The model under review builds one solid part; all positions refer to its coordinate system, in mm. A direction names the side the tool comes from. Round coordinates to 2 decimals unless told otherwise and drop trailing zeros. Order: outer loops, then holes, each group sorted by start corner. A loop starts at its lowest first (then second) coordinate and runs counter-clockwise, first axis right, second up. Notation, with made-up numbers: M -35.5,35.5 L 7.5,35.5 A15 cw 7.5,58.5 Z; hole C 83.25,86 d8. An arc over 180 degrees is marked long. One line per item, written item: value. Start each with the question number.
Autodesk Inventor part; units mm, degrees
ref_plane "YZ Plane" through (0, 0, 0) normal (1, 0, 0) x (0, 1, 0)
ref_plane "XZ Plane" through (0, 0, 0) normal (0, 1, 0) x (-1, 0, 0)
ref_plane "XY Plane" through (0, 0, 0) normal (0, 0, 1) x (1, 0, 0)
sketch "Sketch1" plane through (0, 0, 0) normal (1, 0, 0) x (0, 1, 0)
  line L0 (15.7193, -14.4333) -> (-9.6807, -14.4333)
  line L1 (-9.6807, -14.4333) -> (-9.6807, 10.9667)
  line L2 (-9.6807, 10.9667) -> (15.7193, 10.9667)
  line L3 (15.7193, 10.9667) -> (15.7193, -14.4333)
  line L4 (15.7193, -14.4333) -> (-9.6807, 10.9667) construction
  line L5 (-9.6807, -14.4333) -> (15.7193, 10.9667) construction
  point P0 (0, 0)
  point P1 (3.0193, -1.7333)
  dimension "d0" = 25.4
  dimension "d1" = 25.4
extrude "Extrusion1" add sketch "Sketch1" along normal blind 25.4
sketch "Sketch2" plane through (0, -9.6807, 10.9667) normal (0, 0, 1) x (1, 0, 0)
  circle A0 centre (12.7, 12.7) radius 2.3749
  point P0 (0, 9.6807)
  dimension "d4" = 4.7498
sketch "Sketch3" plane through (0, -9.6807, 10.9667) normal (0, 0, 1) x (1, 0, 0)
  line L0 (0, 0) -> (0, 25.4)
  line L1 (0, 0) -> (25.4, 0)
  line L2 (25.4, 25.4) -> (25.4, 0)
  line L3 (0, 25.4) -> (25.4, 25.4)
  point P0 (0, 9.6807)
extrude "Extrusion2" cut sketch "Sketch2" against normal blind 1.27
sketch "Sketch4" plane through (0, 15.7193, 10.9667) normal (0, 1, 0) x (1, 0, 0)
  circle A0 centre (6.3453, 19.0547) radius 2.3749
  circle A1 centre (12.7, 12.7) radius 2.3749
  circle A2 centre (19.0547, 6.3453) radius 2.3749
  point P0 (0, 10.9667)
  dimension "d7" = 4.7498
  dimension "d8" = 4.7498
  dimension "d9" = 4.7498
extrude "Extrusion3" cut sketch "Sketch4" against normal blind 1.27
sketch "Sketch5" plane through (0, -9.6807, -14.4333) normal (0, -1, 0) x (1, 0, 0)
  circle A0 centre (6.3453, 19.0547) radius 2.3749
  circle A1 centre (19.0547, 19.0547) radius 2.3749
  circle A2 centre (6.3453, 6.3453) radius 2.3749
  circle A3 centre (19.0547, 6.3453) radius 2.3749
  point P0 (0, 14.4333)
  dimension "d12" = 4.7498
  dimension "d13" = 4.7498
  dimension "d14" = 4.7498
  dimension "d15" = 4.7498
extrude "Extrusion4" cut sketch "Sketch5" against normal blind 1.27
sketch "Sketch6" plane through (0, -9.6807, -14.4333) normal (0, 0, -1) x (-1, 0, 0)
  circle A0 centre (-19.0556, 19.0556) radius 2.3749
  circle A1 centre (-6.3444, 19.0556) radius 2.3749
  circle A2 centre (-6.3444, 6.3444) radius 2.3749
  circle A3 centre (-19.0556, 6.3444) radius 2.3749
  circle A4 centre (-6.3444, 12.7) radius 2.3749
  circle A5 centre (-19.0556, 12.7) radius 2.3749
  point P0 (0, 9.6807)
  dimension "d18" = 4.7498
  dimension "d19" = 4.7498
  dimension "d20" = 4.7498
  dimension "d21" = 4.7498
  dimension "d22" = 4.7498
  dimension "d23" = 4.7498
extrude "Extrusion5" cut sketch "Sketch6" against normal blind 1.27
sketch "Sketch7" plane through (0, 0, 0) normal (-1, 0, 0) x (0, 0, 1)
  line L0 (-14.4333, 15.7193) -> (-14.4333, -9.6807)
  line L1 (-14.4333, -9.6807) -> (10.9667, -9.6807)
  line L2 (10.9667, -9.6807) -> (10.9667, 15.7193)
  line L3 (10.9667, 15.7193) -> (-14.4333, 15.7193)
  circle A0 centre (-8.0833, 9.3693) radius 2.3749
  circle A1 centre (4.6222, 9.3693) radius 2.3749
  circle A2 centre (4.6222, -3.3307) radius 2.3749
  circle A3 centre (-8.0833, -3.3307) radius 2.3749
  circle A4 centre (-1.7333, 3.0193) radius 2.3749
  point P0 (0, 0)
  dimension "d26" = 6.35
  dimension "d27" = 6.35
  dimension "d28" = 6.35
  dimension "d29" = 6.3444
  dimension "d30" = 6.35
  dimension "d31" = 6.3444
  dimension "d32" = 6.35
  dimension "d33" = 6.35
  dimension "d34" = 12.7
  dimension "d35" = 12.7
  dimension "d36" = 4.7498
  dimension "d37" = 4.7498
  dimension "d38" = 4.7498
  dimension "d39" = 4.7498
  dimension "d40" = 4.7498
extrude "Extrusion6" cut sketch "Sketch7" against normal blind 1.27 contours A0 | A1 | A2 | A3 | A4
sketch "Sketch8" plane through (25.4, 0, 0) normal (1, 0, 0) x (0, 0, -1)
  line L0 (14.4333, -9.6807) -> (14.4333, 15.7193)
  line L1 (14.4333, 15.7193) -> (-10.9667, 15.7193)
  line L2 (-10.9667, 15.7193) -> (-10.9667, -9.6807)
  line L3 (-10.9667, -9.6807) -> (14.4333, -9.6807)
  circle A0 centre (-4.6167, 9.3693) radius 2.3749
  circle A1 centre (8.0833, -3.3307) radius 2.3749
  point P0 (0, 0)
  dimension "d43" = 4.7498
  dimension "d44" = 4.7498
  dimension "d45" = 6.35
  dimension "d46" = 6.35
  dimension "d47" = 6.35
  dimension "d48" = 6.35
extrude "Extrusion7" cut sketch "Sketch8" against normal blind 1.27 contours A0 | A1
fillet "Fillet1" radius 2.54 11 edges at (12.7, 15.7193, 10.9667) (0, 3.0193, 10.9667) (25.4, 3.0193, 10.9667) (25.4, 15.7193, -1.7333) (12.7, 15.7193, -14.4333) (0, 15.7193, -1.7333) (0, -9.6807, -1.7333) (0, 3.0193, -14.4333) (25.4, -9.6807, -1.7333) (12.7, -9.6807, -14.4333) (25.4, 3.0193, -14.4333)
fillet "Fillet2" radius 2.54 3 edges at (24.6561, -8.9367, 10.2227) (0.7439, -8.9367, 10.2227) (12.7, -9.6807, 10.9667)
properties part number "Goldnsilver die"
Item 1: Clearance check with flat-ended pins moving along their axes: P1, Ø1.4, axis at x = 18.5, y = 9, coming from the -Z side; P2, Ø1.4, axis at x = 5.5, z = 4, coming from the -Y side; P3, Ø1.4, axis at y = 10.5, z = 4, coming from the +X side; P4, Ø10, axis at y = 11.5, z = -9, coming from the -X side. State where each tip first meets the part, or that it passes through.
Item 2: Consider section D-D, the plane z = -2.25. Give the boundary of the cut face in (x, y), then the cut area to 3 significant figures.
Item 3: Consider section A-A, the plane x = 12.7. Give the boundary of the cut face in (y, z).
Item 4: The part is to be moulded in two halves that separate along X. For faces 5 (the cylindrical face through (21.25, 15.09, 5.53)), 6 (the cylindrical face through (0.626, 10.083, -5.818)), 7 (the flat face through (1.27, -3, 5)), 8 (the cylindrical face through (24.636, 2.877, -13.709)), say which applies: pulls with the +X half, pulls with the -X half, needs draft (parallel to the pull), parting line crosses it, or undercut.
Item 5: Wall thickness on L1, parallel to Z at x = 23, y = 2.25; L2, parallel to Z at x = 4.25, y = -2.75; L3, parallel to X at y = 11.5, z = -7.5: over which ranges is each line inside the solid? List them lowest first.
Item 6: Machinability: for faces 1 (the flat face through (24.13, 9, 5)), 2 (the cylindrical face through (4.08, 10.09, -13.81)), 3 (the flat face through (1.27, 3, -2)), 4 (the flat face through (6, -8.411, 5)), which of the approach directions +Z, -Z, +X, -X, +Y, -Y give a long, thin tool a straight path to every point of the face, cutting with its end or side? Answer none if there is none.
Computed:
1. P1: stops at z = -13.16
1. P2: stops at y = -8.41
1. P3: stops at x = 24.13
1. P4: stops at x = 0
2. outline: M 0,-7.14 A2.54 ccw 2.54,-9.68 L 22.86,-9.68 A2.54 ccw 25.4,-7.14 L 25.4,13.18 A2.54 ccw 22.86,15.72 L 15.02,15.72 L 15.02,14.45 L 10.38,14.45 L 10.38,15.72 L 2.54,15.72 A2.54 ccw 0,13.18 L 0,5.34 L 1.27,5.34 L 1.27,0.7 L 0,0.7 Z
2. area: 628 mm^2
3. outline: M -9.68,-11.89 A2.54 ccw -7.14,-14.43 L 13.18,-14.43 A2.54 ccw 15.72,-11.89 L 15.72,-4.11 L 14.45,-4.11 L 14.45,0.64 L 15.72,0.64 L 15.72,8.43 A2.54 ccw 13.18,10.97 L 5.39,10.97 L 5.39,9.7 L 0.64,9.7 L 0.64,10.97 L -7.14,10.97 A2.54 ccw -9.68,8.43 Z
4. face 5: undercut
4. face 6: needs draft
4. face 7: pulls with the -X half
4. face 8: pulls with the +X half
5. L1: z = -14.43 to 10.96
5. L2: z = -13.16 to 10.97
5. L3: x = 1.27 to 25.4
6. face 1: +X
6. face 2: -Z
6. face 3: -X
6. face 4: -Y
